Geometry check sheet. Reference: the model listing, model coordinates, mm. A direction names the side the tool comes from. Give positions to 0.01 mm unless a question says otherwise; leave off trailing zeros. Write each loop counter-clockwise with the first axis right and the second up, starting at its lowest first coordinate (ties: lowest second). Pieces come first, ordered by that corner, then holes. Notation, with made-up numbers: (23, -21.5) -> (40, -21.5) arc R24 cw to (40, -0.5) -> close; hole circle Ø6 at (-25, 27). An arc over 180 degrees is marked (long way). Use a Markdown table: item, result. Add a question column.
Autodesk Fusion 360 part; units mm, degrees
sketch "Sketch1" plane through (0, 0, 0) normal (0, 0, 1) x (1, 0, 0)
  line L0 (3.5, 81.3196) -> (3.5, -80.4746) construction
  line L1 (55.75, 77.2981) -> (-48.75, 77.2981)
  line L2 (-48.75, 77.2981) -> (-48.75, -2.2019)
  line L3 (-48.75, -2.2019) -> (55.75, -2.2019)
  line L4 (55.75, -2.2019) -> (55.75, 77.2981)
  line L5 (55.75, 77.2981) -> (-48.75, -2.2019) construction
  line L6 (-48.75, 77.2981) -> (55.75, -2.2019) construction
  line L7 (-44, -6.2019) -> (51, -6.2019)
  line L8 (51, -6.2019) -> (51, -67.2019)
  line L9 (51, -67.2019) -> (-44, -67.2019)
  line L10 (-44, -67.2019) -> (-44, -6.2019)
  line L11 (-44, -6.2019) -> (51, -67.2019) construction
  line L12 (51, -6.2019) -> (-44, -67.2019) construction
  line L13 (-42.5, 76.5481) -> (49.5, 76.5481)
  line L14 (49.5, 76.5481) -> (49.5, -1.4519)
  line L15 (49.5, -1.4519) -> (-42.5, -1.4519)
  line L16 (-42.5, -1.4519) -> (-42.5, 76.5481)
  line L17 (-42.5, 76.5481) -> (49.5, -1.4519) construction
  line L18 (49.5, 76.5481) -> (-42.5, -1.4519) construction
  line L19 (57, -6.2019) -> (-50, -6.2019)
  line L20 (-50, -6.2019) -> (-50, -67.2019)
  line L21 (-50, -67.2019) -> (57, -67.2019)
  line L22 (57, -67.2019) -> (57, -6.2019)
  line L23 (57, -6.2019) -> (-50, -67.2019) construction
  line L24 (-50, -6.2019) -> (57, -67.2019) construction
  line L25 (-209.3085, -13.7554) -> (162.3486, -13.7554) construction
  line L26 (58.75, -74.2019) -> (-51.75, -74.2019)
  line L27 (-51.75, -74.2019) -> (-51.75, 84.2981)
  line L28 (-51.75, 84.2981) -> (58.75, 84.2981)
  line L29 (58.75, 84.2981) -> (58.75, -74.2019)
  line L30 (58.75, -74.2019) -> (-51.75, 84.2981) construction
  line L31 (-51.75, -74.2019) -> (58.75, 84.2981) construction
  line L32 (-9.9758, -6.2019) -> (23.4575, -6.2019)
  line L33 (23.4575, -6.2019) -> (23.4575, -1.4519)
  line L34 (23.4575, -1.4519) -> (-9.9758, -1.4519)
  line L35 (-9.9758, -1.4519) -> (-9.9758, -6.2019)
  point P0 (3.5, 37.5481)
  point P1 (3.5, -36.7019)
  point P2 (3.5, 37.5481)
  point P3 (3.5, -36.7019)
  point P4 (3.5, 5.0481)
  dimension "d11" = 104.5
  dimension "d12" = 79.5
  dimension "d13" = 95
  dimension "d14" = 61
  dimension "d15" = 92
  dimension "d16" = 78
  dimension "d17" = 107
  dimension "d18" = 61
  dimension "d19" = 74.25
  dimension "d21" = 110.5
  dimension "d22" = 158.5
  dimension "d23" = 7
extrude "Extrude1" add sketch "Sketch1" along normal blind 2 contours L1 L2 L3 L4 L13 L14 L15 L16 L33 L35 | L3 L7 L19 L32 L33 L35 | L3 L15 L33 L34 L35 | L8 L19 L21 L22 | L10 L19 L20 L21 | L26 L27 L28 L29
extrude "Extrude2" add sketch "Sketch1" against normal blind 10
extrude "Extrude3" add sketch "Sketch1" against normal blind 3 contours L3 L7 L19 L32 L33 L35
equation "screenWidth = 92 mm"
equation "screenHeight = 78 mm"
equation "solarWidth = 107 mm"
equation "solarHeight = 61 mm"
equation "solarBoardWidth = 95 mm"
equation "solarBoardOHeight = solarHeight"
equation "screenBoardWidth = 104.5 mm"
equation "screenBoardHeight = 79.5 mm"
equation "middleSpace = 4 mm"
equation "border = 3 mm"
equation "d11 = screenBoardWidth"
equation "d12 = screenBoardHeight"
equation "d13 = solarBoardWidth"
equation "d14 = solarBoardOHeight"
equation "d15 = screenWidth"
equation "d16 = screenHeight"
equation "d17 = solarWidth"
equation "d18 = solarHeight"
equation "d19 = ( ( screenBoardHeight + solarBoardOHeight ) / 2 ) + middleSpace"
equation "boardThickness = 10 mm"
equation "d21 = screenBoardWidth + ( border * 2 )"
equation "d22 = solarBoardOHeight + screenBoardHeight + middleSpace + ( borderTop * 2 )"
equation "d23 = borderTop"
equation "faceThickness = 2 mm"
equation "d25 = faceThickness"
equation "borderTop = 7 mm"
1) Gauge pin test, flat end, axial feed: P1, Ø6.5, axis at x = -45.5, y = -47, coming from the -Z side. Record the tip position at first contact, or that the pin passes through.
2) Sectioned sample at D-D, the plane y = 7. Enter the section's corners in (x, z).
3) Tool access check on faces 1 (the face through (-51.75, 4, -4)), 2 (the face through (57, -37, -5)). Record the directions out of +Z, -Z, +X, -X, +Y, -Y that give a thin tool (end or side, any length) a straight path to the whole face; none if there is none.
4) Sectioned sample at C-C, the plane y = -15.5. Enter the section's corners in (x, z), and give its area (3 significant figures).
5) Draft check along Y on faces 3 (the face through (3, -67.202, -4)), 4 (the face through (23.458, -4, -6)), 5 (the face through (4, -74.202, -4)), 6 (the face through (58.75, 6, -4)). Enter one of: +Y half, -Y half, draft (parallel to the pull), parting line (faces both ways), or undercut.
6) Material ranges on probe 1 along Y at (x, z) = (45, -8.75); probe 2 along Y at (x, z) = (-12, 1.25); probe 3 along X at (y, z) = (-13, -9.25), recorded low to high. Write a range as [from, to].
7) Sectioned sample at A-A, the plane z = -7. Enter the section's corners in (x, y), and give its area (3 significant figures).
8) Sectioned sample at B-B, the plane x = 36.5. Enter the section's corners in (y, z).
Check values:
| question | item | result |
|---|---|---|
| 1 | P1 | z = 0 |
| 2 | outline | (-51.75, -10) -> (-48.75, -10) -> (-48.75, 0) -> (-42.5, 0) -> (-42.5, 2) -> (-51.75, 2) -> close; (49.5, 0) -> (55.75, 0) -> (55.75, -10) -> (58.75, -10) -> (58.75, 2) -> (49.5, 2) -> close |
| 3 | face 1 | +Z, -Z, -X, +Y, -Y |
| 3 | face 2 | -Z |
| 4 | outline | (-51.75, -10) -> (-50, -10) -> (-50, 0) -> (-44, 0) -> (-44, 2) -> (-51.75, 2) -> close; (51, 0) -> (57, 0) -> (57, -10) -> (58.75, -10) -> (58.75, 2) -> (51, 2) -> close |
| 4 | area | 66.0 mm² |
| 5 | face 3 | undercut |
| 5 | face 4 | undercut |
| 5 | face 5 | -Y half |
| 5 | face 6 | draft |
| 6 | probe 1 | [-74.2, -67.2], [-6.2, -2.2], [77.3, 84.3] |
| 6 | probe 2 | [-74.2, -67.2], [-6.2, -1.45], [76.55, 84.3] |
| 6 | probe 3 | [-51.75, -50], [57, 58.75] |
| 7 | outline | (-51.75, -74.2) -> (58.75, -74.2) -> (58.75, 84.3) -> (-51.75, 84.3) -> close; hole (-50, -67.2) -> (57, -67.2) -> (57, -6.2) -> (23.46, -6.2) -> (23.46, -2.2) -> (55.75, -2.2) -> (55.75, 77.3) -> (-48.75, 77.3) -> (-48.75, -2.2) -> (-9.98, -2.2) -> (-9.98, -6.2) -> (-50, -6.2) -> close |
| 7 | area | 2,550 mm² |
| 8 | outline | (-74.2, -10) -> (-67.2, -10) -> (-67.2, 2) -> (-74.2, 2) -> close; (-6.2, -10) -> (-2.2, -10) -> (-2.2, 0) -> (-1.45, 0) -> (-1.45, 2) -> (-6.2, 2) -> close; (76.55, 0) -> (77.3, 0) -> (77.3, -10) -> (84.3, -10) -> (84.3, 2) -> (76.55, 2) -> close |
